from build123d import *

# Parameters (mm, degrees)
SKETCH1_R           = 4
BOSS_EXTRUDE1_DEPTH = 1
SKETCH3_R           = 4.75
BOSS_EXTRUDE3_DEPTH = 1
SKETCH4_R           = 1
CUT_EXTRUDE1_DEPTH  = 8.818247886


with BuildPart() as part:
    # Sketch1 → Boss-Extrude1 (new, symmetric)
    with BuildSketch(Plane.XY):
        Circle(SKETCH1_R)
    extrude(amount=BOSS_EXTRUDE1_DEPTH, both=True)

    # Sketch3 → Boss-Extrude3 (add)
    with BuildSketch(Plane.XY.offset(1)):
        Circle(SKETCH3_R)
    boss_extrude3 = extrude(amount=BOSS_EXTRUDE3_DEPTH)

    # Mirror1: Boss-Extrude3 across plane
    add(boss_extrude3.mirror(Plane.XY))

    # Sketch4 → Cut-Extrude1 (cut, through all)
    with BuildSketch(Plane.XY.offset(2)):
        Circle(SKETCH4_R)
    extrude(amount=-CUT_EXTRUDE1_DEPTH, mode=Mode.SUBTRACT)


solid = part.part
Model file for the job. Use its own axes, mm. A direction names the side the tool comes from. Coordinates: 2 decimals unless noted, no trailing zeros. Write each loop counter-clockwise with the first axis right and the second up, starting at its lowest first coordinate (ties: lowest second). Pieces come first, ordered by that corner, then holes. Notation, with made-up numbers: (-23, 38.5) -> (-6, 38.5) arc R18 cw to (-6, 44.5) -> close; hole circle Ø2 at (25.5, 28). An arc over 180 degrees is marked (long way). One line per item, written item: value. Start each with the question number.
1) Slice it at C-C on z = 1.15. Write the cut outline in (x, y).
2) Slice it at A-A on x = 0. Write the cut outline in (y, z).
3) Pull direction Z, two halves, no side cores. Call faces 3 (the face through (-0.867, -3.905, 0.014)), 4 (the face through (0, -1, 0)), 5 (the face through (1, -1, -2)), 6 (the face through (-4, -2, -1)): +Z half, -Z half, draft (parallel to the pull), parting line (faces both ways), or undercut.
4) Slice it at D-D on y = 3.25. Write the cut outline in (x, z), then the cut area to 3 significant figures.
5) Which spindle directions (+Z, -Z, +X, -X, +Y, -Y) get a long thin tool onto all of the face, cutting with end or side? Do faces 1 (the face through (-4, -2, 1)), 2 (the face through (2.192, -4.214, 1.493)). Say none if no direction does.
6) Flat gauge pins, fed straight in: pin 1 Ø1.6 at (x, y) = (0, 0) entering from +Z; pin 2 Ø1.5 at (y, z) = (-1.5, -1.5) entering from -X. Where does each tip first touch, or does it go through?
7) Probe probe 1 along Y at (x, z) = (0, -0.25); probe 2 along Y at (x, z) = (0, -1.2); probe 3 along Z at (x, y) = (0.75, 4). List the from-to ranges inside material, lowest first.
Answers follow:
1. outline: circle Ø9.5 at (0, 0); hole circle Ø2 at (0, 0)
2. outline: (-4.75, -2) -> (-1, -2) -> (-1, 2) -> (-4.75, 2) -> (-4.75, 1) -> (-4, 1) -> (-4, -1) -> (-4.75, -1) -> close; (1, -2) -> (4.75, -2) -> (4.75, -1) -> (4, -1) -> (4, 1) -> (4.75, 1) -> (4.75, 2) -> (1, 2) -> close
3. face 3: undercut
3. face 4: draft
3. face 5: -Z half
3. face 6: undercut
4. outline: (-3.46, -2) -> (3.46, -2) -> (3.46, -1) -> (2.33, -1) -> (2.33, 1) -> (3.46, 1) -> (3.46, 2) -> (-3.46, 2) -> (-3.46, 1) -> (-2.33, 1) -> (-2.33, -1) -> (-3.46, -1) -> close
4. area: 23.2 mm2
5. face 1: none
5. face 2: +Z, -Z
6. pin 1: through
6. pin 2: x = -4.69
7. probe 1: -4 to -1, 1 to 4
7. probe 2: -4.75 to -1, 1 to 4.75
7. probe 3: -2 to -1, 1 to 2
